Here's the drawing with two shaded views (mm, measured from the low corner). I have some questions. A direction names the side the tool comes from. Coordinates: 2 decimals unless noted, no trailing zeros. Loops run counter-clockwise (first coordinate to the right, second up) from the corner with the lowest first, then second, coordinate; pieces in that order, holes last. Notation, with made-up numbers: (67.5, 24) -> (93.5, 24) arc R22 cw to (93.5, 50) -> close; hole circle Ø4 at (12, -15). An arc over 180 degrees is marked (long way). Answer as a JSON object with one key per item and string values. Group by question number.
1) I want a section at B-B (y = 2.25). Write out the boundary of the cut face in (x, z).
2) If we mould it in two halves opening along X, with no side actions, what happens to the marked faces 4, 5 and 6? For each: +X half, -X half, draft (parallel to the pull), parting line (faces both ways), or undercut.
3) I'm going to push flat-ended pins straight in: pin 1 (0.6 mm diameter, centred on x = 0.5, z = 1, fed in from +Y) (1 decimal); pin 2 (0.5 mm diameter, centred on x = 4.5, z = 1, fed in from -Y); pin 3 (0.6 mm diameter, centred on y = 3, z = 1, fed in from -X). Where does each tip first touch, or does it pass through?
4) I want a section at C-C (y = 8.75). Write out the boundary of the cut face in (x, z).
5) I want a section at A-A (z = 0.85). Write out the boundary of the cut face in (x, y).
6) I need wall thicknesses on probe 1 along X at (y, z) = (16.5, 1.9); probe 2 along Y at (x, z) = (5.2, 1.7); probe 3 along X at (y, z) = (4.5, 0.85). Which ranges of each line are inside material? Lowest first, please. Write a range as [from, to].
7) Which directions (+Z, -Z, +X, -X, +Y, -Y) give clear straight access to the entire face, cutting with the end or side of a thin tool? Please do the marked faces 1, 2 and 3.
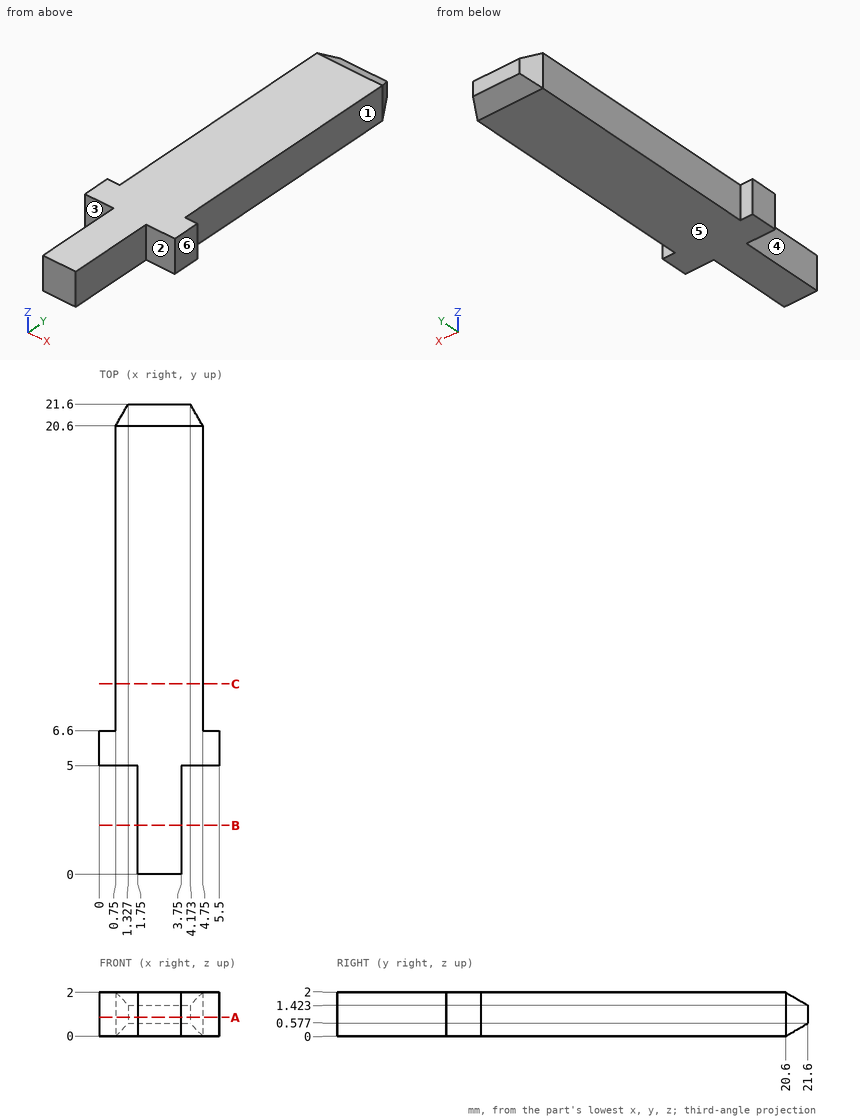
Determined:
{
 "1": {"outline": "(1.75, 0) -> (3.75, 0) -> (3.75, 2) -> (1.75, 2) -> close"},
 "2": {"face 4": "-X half", "face 5": "draft", "face 6": "+X half"},
 "3": {"pin 1": "y = 20.7", "pin 2": "y = 5", "pin 3": "x = 1.75"},
 "4": {"outline": "(0.75, 0) -> (4.75, 0) -> (4.75, 2) -> (0.75, 2) -> close"},
 "5": {"outline": "(0, 5) -> (1.75, 5) -> (1.75, 0) -> (3.75, 0) -> (3.75, 5) -> (5.5, 5) -> (5.5, 6.6) -> (4.75, 6.6) -> (4.75, 20.6) -> (4.17, 21.6) -> (1.33, 21.6) -> (0.75, 20.6) -> (0.75, 6.6) -> (0, 6.6) -> close"},
 "6": {"probe 1": "[0.75, 4.75]", "probe 2": "[5, 6.6]", "probe 3": "[1.75, 3.75]"},
 "7": {"face 1": "+Z, -Z, +X, +Y", "face 2": "+Z, -Z, +X, -Y", "face 3": "+Z, -Z, -X, -Y"}
}
